Geometry check sheet. Reference: drawing and pictorial views, mm from the part's lowest x, y, z. Coordinates: 2 decimals unless noted, no trailing zeros. Loops run counter-clockwise (first coordinate to the right, second up) from the corner with the lowest first, then second, coordinate; pieces in that order, holes last.
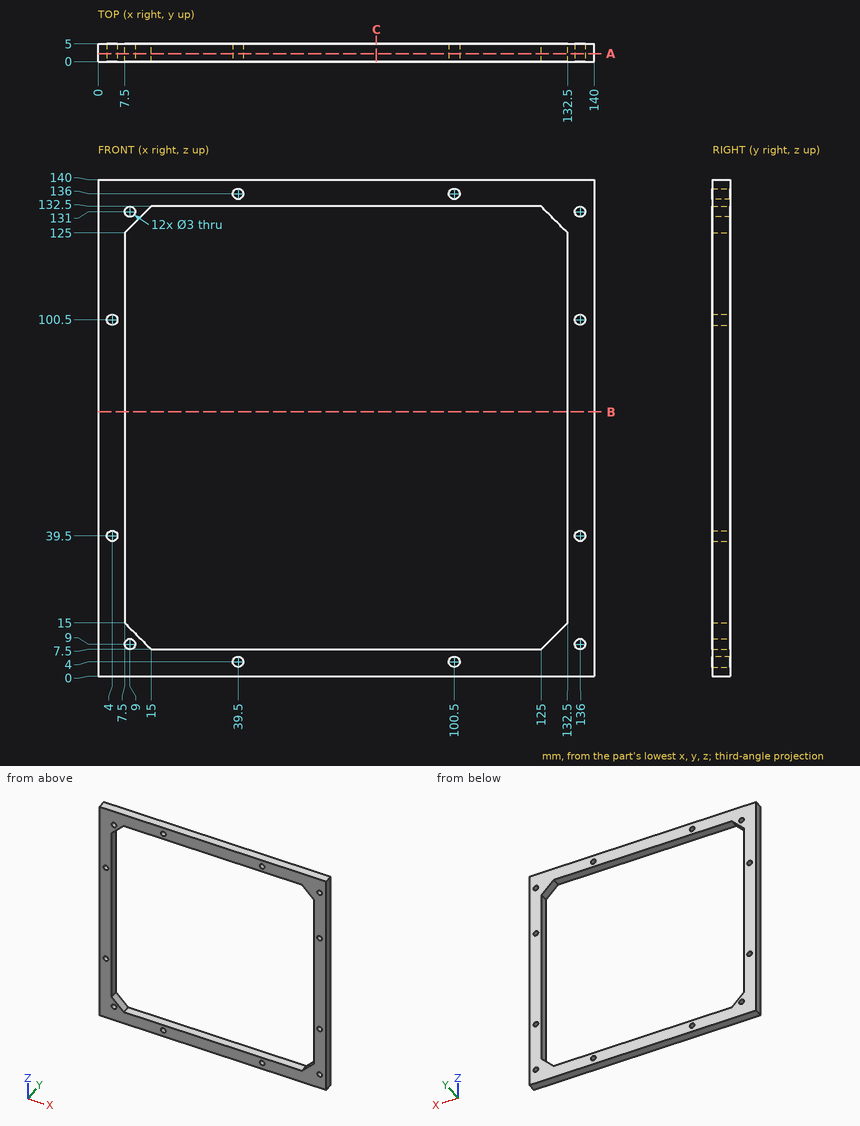
1) Section check A-A on y = 2.3. Count the separate pieces of the cut face and the enclosed holes in it, and give its area (3 significant figures).
Data:
separate pieces: 1
enclosed holes: 13
area: 4,000 mm2
2) Section check B-B on z = 74.5. Record the cut outline in (x, y).
Data:
outline: (0, 0) - (7.5, 0) - (7.5, 5) - (0, 5) - close; (132.5, 0) - (140, 0) - (140, 5) - (132.5, 5) - close
3) Section check C-C on x = 78.5. Record the cut outline in (y, z).
Data:
outline: (0, 0) - (5, 0) - (5, 7.5) - (0, 7.5) - close; (0, 132.5) - (5, 132.5) - (5, 140) - (0, 140) - close
4) Material ranges on probe 1 along X at (y, z) = (3.1, 136); probe 2 along Z at (x, y) = (136, 1.75); probe 3 along X at (y, z) = (3.55, 39.5), recorded low to high.
Data:
probe 1: x = 0 to 38, 41 to 99, 102 to 140
probe 2: z = 0 to 7.5, 10.5 to 38, 41 to 99, 102 to 129.5, 132.5 to 140
probe 3: x = 0 to 2.5, 5.5 to 7.5, 132.5 to 134.5, 137.5 to 140
